from build123d import *

# Parameters (mm, degrees)
SKETCH1_W                           = 60
SKETCH1_H                           = 60
BOSS_EXTRUDE1_DEPTH                 = 10
SKETCH2_R                           = 6
CUT_EXTRUDE1_DEPTH                  = 10
SKETCH3_R                           = 19.05
CUT_EXTRUDE2_DEPTH                  = 1.5
SKETCH4_R                           = 2.25
CUT_EXTRUDE3_DEPTH                  = 10
F_4_5_4_5_DIAMETER_HOLE1_AT_2_COUNT = 2
F_4_5_4_5_DIAMETER_HOLE1_AT_2_PITCH = 30.150470286
F_4_5_4_5_DIAMETER_HOLE1_AT_3_COUNT = 2
F_4_5_4_5_DIAMETER_HOLE1_AT_3_PITCH = 21.319601995
F_4_5_4_5_DIAMETER_HOLE1_AT_4_COUNT = 2
F_4_5_4_5_DIAMETER_HOLE1_AT_4_PITCH = 21.319601995
SKETCH6_R                           = 22.4
CUT_EXTRUDE4_DEPTH                  = 3


with BuildPart() as part:
    # Sketch1 → Boss-Extrude1 (new body)
    with BuildSketch(Plane.XY):
        Rectangle(SKETCH1_W, SKETCH1_H)
    extrude(amount=BOSS_EXTRUDE1_DEPTH)

    # Sketch2 → Cut-Extrude1 (cut)
    with BuildSketch(Plane.XY.offset(10)):
        Circle(SKETCH2_R)
    extrude(amount=-CUT_EXTRUDE1_DEPTH, mode=Mode.SUBTRACT)

    # Sketch3 → Cut-Extrude2 (cut)
    with BuildSketch(Plane.XY.offset(10)):
        Circle(SKETCH3_R)
    extrude(amount=-CUT_EXTRUDE2_DEPTH, mode=Mode.SUBTRACT)

    # Sketch4 → Cut-Extrude3 (cut)
    with BuildSketch(Plane.XY.offset(10)):
        with Locations((-23.57, 23.57)):
            Circle(SKETCH4_R)
        with Locations((23.57, 23.57)):
            Circle(SKETCH4_R)
        with Locations((23.57, -23.57)):
            Circle(SKETCH4_R)
        with Locations((-23.57, -23.57)):
            Circle(SKETCH4_R)
    extrude(amount=-CUT_EXTRUDE3_DEPTH, mode=Mode.SUBTRACT)

    # Sketch5 → Ø4.5 (4.5) Diameter Hole1 (revolve, cut)
    with BuildSketch(Plane(origin=(-15.075188443, 0.037523467, 8.5), x_dir=(0, -1, 0), z_dir=(1, 0, 0))):
        Polygon((0, 0), (0, 16.351936393), (2.25, 15), (2.25, 2.75), (5, 0), align=None)
    f_4_5_4_5_diameter_hole1 = revolve(axis=Axis((-15.075188443, 0.037523467, 14.85), (0, 0, -1)), mode=Mode.SUBTRACT)

    # Ø4.5 (4.5) Diameter Hole1 at 2: Ø4.5 (4.5) Diameter Hole1 ×2
    with Locations(*[Vector(0.9999969022354874, -0.0024890800366937364, 0) * (i * F_4_5_4_5_DIAMETER_HOLE1_AT_2_PITCH) for i in range(1, F_4_5_4_5_DIAMETER_HOLE1_AT_2_COUNT)]):
        add(f_4_5_4_5_diameter_hole1, mode=Mode.SUBTRACT)

    # Ø4.5 (4.5) Diameter Hole1 at 3: Ø4.5 (4.5) Diameter Hole1 ×2
    with Locations(*[Vector(0.7088646361091163, 0.705344545363392, 0) * (i * F_4_5_4_5_DIAMETER_HOLE1_AT_3_PITCH) for i in range(1, F_4_5_4_5_DIAMETER_HOLE1_AT_3_COUNT)]):
        add(f_4_5_4_5_diameter_hole1, mode=Mode.SUBTRACT)

    # Ø4.5 (4.5) Diameter Hole1 at 4: Ø4.5 (4.5) Diameter Hole1 ×2
    with Locations(*[Vector(0.705344545363392, -0.7088646361091163, 0) * (i * F_4_5_4_5_DIAMETER_HOLE1_AT_4_PITCH) for i in range(1, F_4_5_4_5_DIAMETER_HOLE1_AT_4_COUNT)]):
        add(f_4_5_4_5_diameter_hole1, mode=Mode.SUBTRACT)

    # Sketch6 → Cut-Extrude4 (cut)
    with BuildSketch(Plane(origin=(0, 0, 0), x_dir=(-1, 0, 0), z_dir=(0, 0, -1))):
        Circle(SKETCH6_R)
    extrude(amount=-CUT_EXTRUDE4_DEPTH, mode=Mode.SUBTRACT)


solid = part.part
Build history of the part. All positions in model axes, mm. A direction names the side the tool comes from. Give positions to 0.01 mm unless a question says otherwise; leave off trailing zeros. Order: outer loops, then holes, each group sorted by start corner. A loop starts at its lowest first (then second) coordinate and runs counter-clockwise, first axis right, second up. Notation, with made-up numbers: M 30,38.5 L 89,38.5 A14 cw 89,63.5 Z; hole C -39.5,-34.5 d7. An arc over 180 degrees is marked long. Put each result on its own line as item: value.
Item 1: Slice it at C-C, the plane z = 4.75. Give the number of separate pieces and of enclosed holes in the cut face, plus the area to 3 significant figures.
From the geometry:
separate pieces: 1
enclosed holes: 9
area: 3,360 mm2
Item 2: Flat gauge pins, fed straight in: pin 1 Ø1.5 at (x, y) = (-19.5, -1.5) entering from -Z; pin 2 Ø6 at (x, y) = (15.08, -0.04) entering from +Z; pin 3 Ø19 at (x, y) = (7, 1.5) entering from +Z. Where does each tip first touch, or does it go through?
From the geometry:
pin 1: stops at z = 3
pin 2: stops at z = 6.51
pin 3: stops at z = 8.5
Item 3: Slice it at D-D, the plane y = -9. Write the cut outline in (x, z).
From the geometry:
outline: M -30,0 L -20.51,0 L -20.51,3 L 20.51,3 L 20.51,0 L 30,0 L 30,10 L 16.79,10 L 16.79,8.5 L -16.79,8.5 L -16.79,10 L -30,10 Z
Item 4: Probe line 1 (Y direction, x = -23.57, z = 5.5); line 2 (X direction, y = 24, z = 2.5). List the from-to ranges inside material, lowest first. Write a range as [from, to].
From the geometry:
line 1: y = [-30, -25.82], [-21.32, 21.32], [25.82, 30]
line 2: x = [-30, -25.78], [-21.36, 21.36], [25.78, 30]
Item 5: 3-axis set-ups, long thin cutter, end or side, ignore diameter. For faces 1 (the flat face through (-4.4, 4.4, 8.5)), 2 (the cylindrical face through (-0.713, -17.221, 4.394)), 3 (the flat face through (-30, 0, 5)), 4 (the cylindrical face through (22.38, 0.98, 1.48)), 5 (the flat face through (0, 19.4, 8.5)): which of +Z, -Z, +X, -X, +Y, -Y reach the whole face in a straight line?
From the geometry:
face 1: +Z
face 2: +Z, -Z
face 3: +Z, -Z, -X, +Y, -Y
face 4: -Z
face 5: none
Item 6: Slice it at A-A, the plane z = 1.25. Write the cut outline in (x, y), plus the area to 3 significant figures.
From the geometry:
outline: M -30,-30 L 30,-30 L 30,30 L -30,30 Z; hole C -23.57,-23.57 d4.5; hole C -23.57,23.57 d4.5; hole C 0,0 d44.8; hole C 23.57,-23.57 d4.5; hole C 23.57,23.57 d4.5
area: 1,960 mm2
Item 7: Two-plate mould, pull along Y, no slides. Class faces 6 (the flat face through (-14, 14, 10)), 7 (the cylindrical face through (-6, 0, 6)): +Y half, -Y half, draft (parallel to the pull), parting line (faces both ways), or undercut.
From the geometry:
face 6: draft
face 7: undercut
Item 8: Slice it at B-B, the plane x = 23.57. Write the cut outline in (y, z).
From the geometry:
outline: M -30,0 L -25.82,0 L -25.82,10 L -30,10 Z; M -21.32,0 L 21.32,0 L 21.32,10 L -21.32,10 Z; M 25.82,0 L 30,0 L 30,10 L 25.82,10 Z
